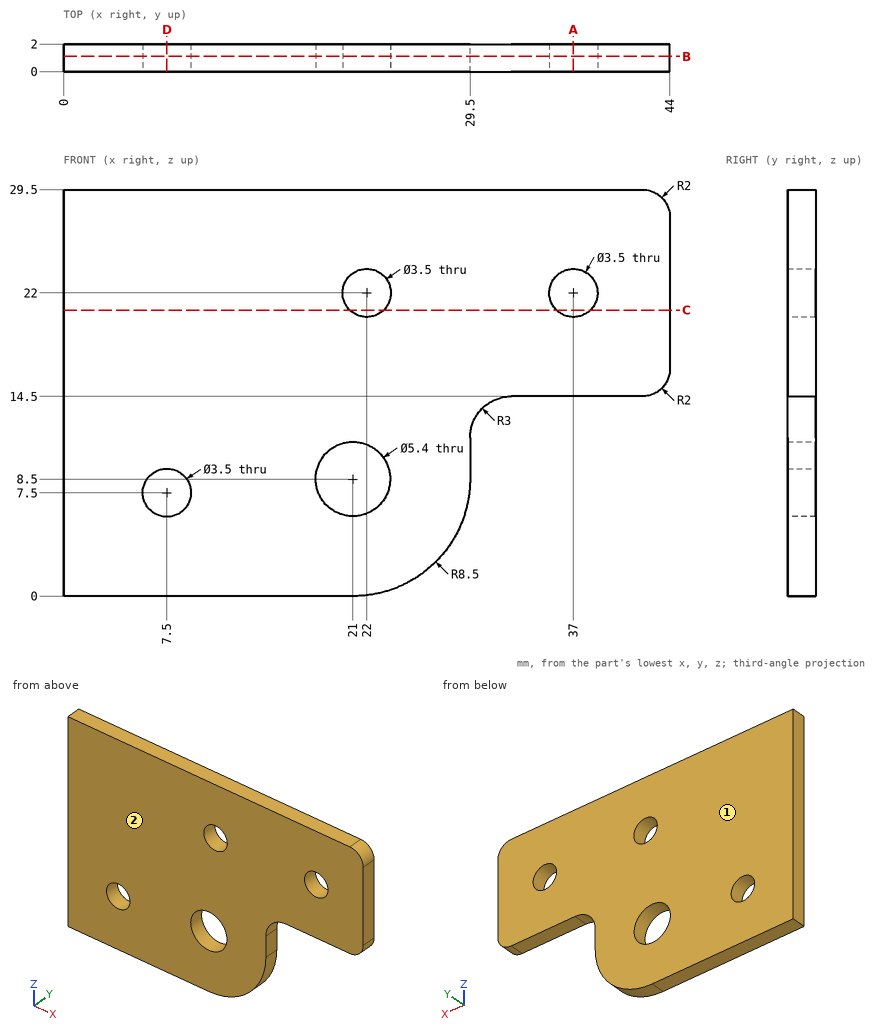
Study the drawing (mm; zero at the part's minimum x, y, z) and answer. Round coordinates to 2 decimals unless told otherwise and drop trailing zeros. Write each loop counter-clockwise with the first axis right and the second up, starting at its lowest first coordinate (ties: lowest second). Pieces come first, ordered by that corner, then holes. Notation, with made-up numbers: (60, 69) - (96, 69) arc R19 ccw to (96, 101) - close; hole circle Ø6 at (78, 77). An arc over 180 degrees is marked (long way). Use a Markdown table: item, result. Add a question column.
1. For a pull along Y with two mould halves and no side action, classify the marked faces 1 and 2 as +Y half, -Y half, draft (parallel to the pull), parting line (faces both ways), or undercut.
2. Consider line 1 (X direction, y = 1.05, z = 7.5); line 2 (X direction, y = 1.8, z = 7) (3 decimals); line 3 (X direction, y = 1.75, z = 11.25). Determine where each line is inside the solid, lowest interval first.
3. The part is cut by section B-B (y = 1.1). Write down the section's boundary in (x, z).
4. The part is cut by section A-A (x = 37). Write down the section's boundary in (y, z), and give its area (3 significant figures).
5. The part is cut by section D-D (x = 7.5). Write down the section's boundary in (y, z), and give its area (3 significant figures).
6. Flat-ended cylindrical pins translate along their axes: P1, Ø2, axis at x = 7.5, z = 7.5, coming from the +Y side; P2, Ø0.6, axis at y = 1, z = 9.5, coming from the +X side. Find the tip coordinate at first contact, or state that the pin passes through.
7. The part is cut by section C-C (z = 20.75). Write down the section's boundary in (x, y), and give its area (3 significant figures).
Reported:
| question | item | result |
|---|---|---|
| 1 | face 1 | +Y half |
| 1 | face 2 | -Y half |
| 2 | line 1 | 0 to 5.75, 9.25 to 18.49, 23.51 to 29.44 |
| 2 | line 2 | 0 to 5.823, 9.177 to 18.755, 23.245 to 29.367 |
| 2 | line 3 | 0 to 29.5 |
| 3 | outline | (0, 0) - (21, 0) arc R8.5 ccw to (29.5, 8.5) - (29.5, 11.5) arc R3 cw to (32.5, 14.5) - (42, 14.5) arc R2 ccw to (44, 16.5) - (44, 27.5) arc R2 ccw to (42, 29.5) - (0, 29.5) - close; hole circle Ø3.5 at (7.5, 7.5); hole circle Ø5.4 at (21, 8.5); hole circle Ø3.5 at (22, 22); hole circle Ø3.5 at (37, 22) |
| 4 | outline | (0, 14.5) - (2, 14.5) - (2, 20.25) - (0, 20.25) - close; (0, 23.75) - (2, 23.75) - (2, 29.5) - (0, 29.5) - close |
| 4 | area | 23.0 mm^2 |
| 5 | outline | (0, 0) - (2, 0) - (2, 5.75) - (0, 5.75) - close; (0, 9.25) - (2, 9.25) - (2, 29.5) - (0, 29.5) - close |
| 5 | area | 52.0 mm^2 |
| 6 | P1 | through |
| 6 | P2 | x = 29.5 |
| 7 | outline | (0, 0) - (20.78, 0) - (20.78, 2) - (0, 2) - close; (23.22, 0) - (35.78, 0) - (35.78, 2) - (23.22, 2) - close; (38.22, 0) - (44, 0) - (44, 2) - (38.22, 2) - close |
| 7 | area | 78.2 mm^2 |
